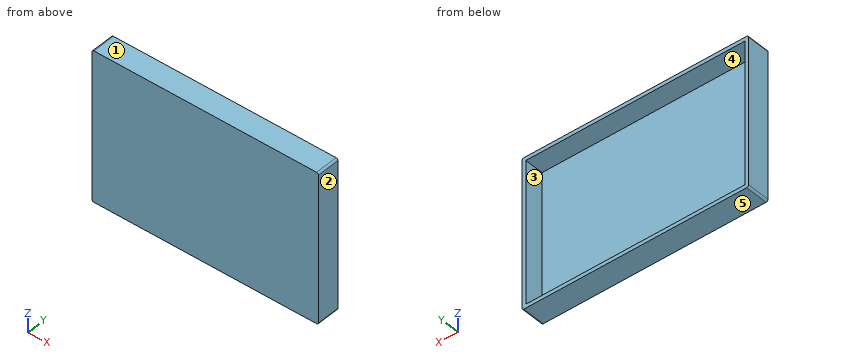
```python
from build123d import *

# Parameters (mm, degrees)
SKETCH1_W           = 115
SKETCH1_H           = 75
BOSS_EXTRUDE1_DEPTH = 10
SHELL1_T            = 2
FILLET1_R           = 1


with BuildPart() as part:
    # Sketch1 → Boss-Extrude1 (new body)
    with BuildSketch(Plane(origin=(0, 0, 0), x_dir=(1, 0, 0), z_dir=(0, 1, 0))):
        Rectangle(SKETCH1_W, SKETCH1_H)
    extrude(amount=BOSS_EXTRUDE1_DEPTH)

    # Shell1
    shell1_openings = [part.faces().sort_by_distance(p)[0] for p in [
        (0, 10, 0),
    ]]
    offset(amount=SHELL1_T, openings=shell1_openings, kind=Kind.INTERSECTION)

    # Fillet1
    # the kernel refuses this fillet: 1 mm, written as the material it takes off along each edge
    with BuildSketch(Plane(origin=(59.5, -4.5, 39.5), x_dir=(-1, 0, 0), z_dir=(0, 1, 0)), Plane(origin=(-59.5, 12.5, 39.5), x_dir=(1, 0, 0), z_dir=(0, -1, 0)), Plane(origin=(-59.5, -4.5, -39.5), x_dir=(1, 0, 0), z_dir=(0, 1, 0)), Plane(origin=(59.5, -4.5, -39.5), x_dir=(0, 0, 1), z_dir=(0, 1, 0))) as fillet1_piece_1:
        with BuildLine():
            CenterArc((FILLET1_R, -FILLET1_R), FILLET1_R, 90, 90)
            Line((0, -FILLET1_R), (0, 0))
            Line((0, 0), (FILLET1_R, 0))
        make_face()
    extrude(amount=17, mode=Mode.SUBTRACT)


solid = part.part
```
Work out the finished part from the listing and answer in its coordinate system (mm). Face numbers are marked on the shaded views. A direction names the side the tool comes from. Give positions to 0.01 mm unless a question says otherwise; leave off trailing zeros. Loops run counter-clockwise (first coordinate to the right, second up) from the corner with the lowest first, then second, coordinate; pieces in that order, holes last. Notation, with made-up numbers: (21, -34.5) -> (29, -34.5) arc R12 ccw to (29, -23.5) -> close; hole circle Ø10 at (37.5, 45.25). An arc over 180 degrees is marked (long way). One line per question, with ' | ' between items. Start each with the question number.
1) Section B-B, the plane x = 5 is taken. Determine the outline of the cut face in (y, z), then the cut area to 3 significant figures.
2) For the marked faces 4 and 5, determine the directions among +Z, -Z, +X, -X, +Y, -Y from which every point of the face is accessible in a straight line to the end or side of a thin tool.
3) Section C-C, the plane z = -13.5 is taken. Determine the outline of the cut face in (x, y), then the cut area to 3 significant figures.
4) Determine the mould class of the marked faces 1, 2 and 3 for opening direction Z: +Z half, -Z half, draft (parallel to the pull), parting line (faces both ways), or undercut.
5) This flat-tipped pin is pushed along its axis until it touches: pin 1 (8 mm diameter, centred on x = -1, z = 27.5, fed in from +Y). Where does it stop, or does it pass through?
6) Section A-A, the plane y = 8 is taken. Determine the outline of the cut face in (x, z), then the cut area to 3 significant figures.
7) Straight lines are drawn through the part: L1, parallel to Z at x = -35, y = 6; L2, parallel to X at y = 6, z = 10; L3, parallel to Y at x = -15, z = -16. For each, find the intervals that lie inside material, in ascending order.
Resolved:
1) outline: (-2, -39.5) -> (10, -39.5) -> (10, -37.5) -> (0, -37.5) -> (0, 37.5) -> (10, 37.5) -> (10, 39.5) -> (-2, 39.5) -> close | area: 198 mm2
2) face 4: +Y | face 5: -Z, +X, -X, +Y, -Y
3) outline: (-59.5, -2) -> (59.5, -2) -> (59.5, 10) -> (57.5, 10) -> (57.5, 0) -> (-57.5, 0) -> (-57.5, 10) -> (-59.5, 10) -> close | area: 278 mm2
4) face 1: +Z half | face 2: draft | face 3: undercut
5) pin 1: y = 0
6) outline: (-59.5, -38.5) arc R1 ccw to (-58.5, -39.5) -> (58.5, -39.5) arc R1 ccw to (59.5, -38.5) -> (59.5, 38.5) arc R1 ccw to (58.5, 39.5) -> (-58.5, 39.5) arc R1 ccw to (-59.5, 38.5) -> close; hole (-57.5, -37.5) -> (57.5, -37.5) -> (57.5, 37.5) -> (-57.5, 37.5) -> close | area: 775 mm2
7) L1: -39.5 to -37.5, 37.5 to 39.5 | L2: -59.5 to -57.5, 57.5 to 59.5 | L3: -2 to 0
